Here's how the part is built. I have some questions about the finished solid (model axes, mm). Face numbers are marked on the shaded views. A direction names the side the tool comes from. Round coordinates to 2 decimals unless told otherwise and drop trailing zeros. Order: outer loops, then holes, each group sorted by start corner. A loop starts at its lowest first (then second) coordinate and runs counter-clockwise, first axis right, second up. Notation, with made-up numbers: (-16, -13) - (0, -13) arc R4 ccw to (0, -8) - close; hole circle Ø4 at (-7, -6.75). An arc over 180 degrees is marked (long way). One line per item, written item: value.
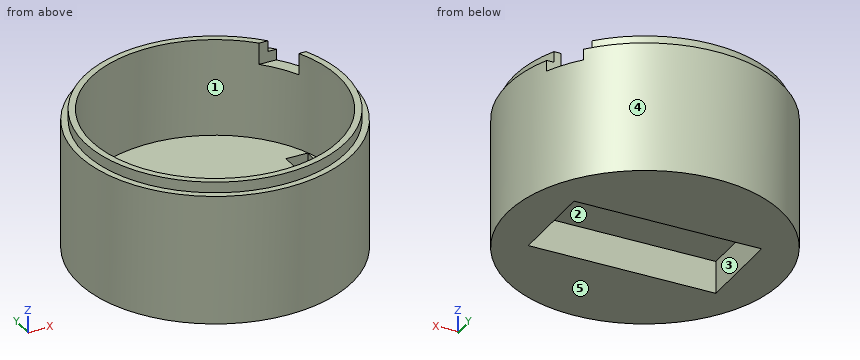
from build123d import *

# Parameters (mm, degrees)
F0_R      = 63
F0_R_2    = 60
F2_DEPTH  = 60
F1_R      = 60
F1_R_2    = 57
F3_DEPTH  = 65
F4_R      = 57
F5_DEPTH  = 60
F7_R      = 57
F8_DEPTH  = 40
F9_W      = 15
F9_H      = 10
F10_DEPTH = 279.5
F11_DEPTH = 71.5
F13_R     = 63
F14_DEPTH = 20
F15_W     = 86
F15_H     = 41
F16_DEPTH = 15
F17_W     = 27.3
F17_H     = 13
F18_DEPTH = 53
F20_DEPTH = 25


# Not quite as in the source:
# - a feature names something its author has since deleted; it is built from what else it names


with BuildPart() as f2:
    # F0 (on Top) → F2 (new body)
    with BuildSketch(Plane.XY):
        Circle(F0_R)
        Circle(F0_R_2, mode=Mode.SUBTRACT)
    extrude(amount=F2_DEPTH)

    # F1 (on Top) → F3 (join)
    with BuildSketch(Plane.XY):
        Circle(F1_R)
        Circle(F1_R_2, mode=Mode.SUBTRACT)
    extrude(amount=F3_DEPTH)

    # F4 (on Top) → F5 (join)
    with BuildSketch(Plane.XY):
        Circle(F4_R)
    extrude(amount=F5_DEPTH)

    # F7 (on offset) → F8 (cut)
    with BuildSketch(Plane.XY.offset(45)):
        Circle(F7_R)
    extrude(amount=-F8_DEPTH, mode=Mode.SUBTRACT)

    # F9 (on Right) → F10 (cut)
    with BuildSketch(Plane.YZ):
        with Locations((32.5, 60)):
            Rectangle(F9_W, F9_H)
    extrude(amount=F10_DEPTH, mode=Mode.SUBTRACT)

    # F1 (on Top) → F11 (cut)
    with BuildSketch(Plane.XY):
        Circle(F1_R_2)
    extrude(amount=F11_DEPTH, mode=Mode.SUBTRACT)

    # F13 (on Top) → F14 (join)
    with BuildSketch(Plane.XY):
        Circle(F13_R)
    extrude(amount=F14_DEPTH)

    # F15 (on Top) → F16 (cut)
    with BuildSketch(Plane.XY):
        Rectangle(F15_W, F15_H)
    extrude(amount=F16_DEPTH, mode=Mode.SUBTRACT)

    # F17 (on Right) → F18 (cut)
    with BuildSketch(Plane.YZ):
        with Locations((6.82, 8.5)):
            Rectangle(F17_W, F17_H)
    extrude(amount=F18_DEPTH, mode=Mode.SUBTRACT)

    # F19 (on offset) → F20 (cut)
    with BuildSketch(Plane.XY.offset(15)):
        Polygon((43, 20.47), (43, 0), (43, -6.83), (53, -6.83), (53, 20.47), align=None)
    extrude(amount=F20_DEPTH, mode=Mode.SUBTRACT)


solid = f2.part
Q1. If we section it at D-D, the plane z = 57: Please give me the cut outline in (x, y) (3 decimals), then the cut area to 3 significant figures.
Results list:
outline: (40.608, 40) - (48.672, 40) arc R63 ccw (long way) to (57.827, 25) - (51.225, 25) arc R57 cw (long way) to start
area: 2,150 mm²
Q2. We'd pull the mould along X, two halves only. Please class the marked faces 3, 4 and 5: released by +X, released by -X, zero draft, split by the parting line, or undercut.
Results list:
face 3: undercut
face 4: split by the parting line
face 5: zero draft
Q3. If we section it at C-C, the plane x = 0: Please give me the cut outline in (y, z).
Results list:
outline: (-63, 0) - (-20.5, 0) - (-20.5, 15) - (20.5, 15) - (20.5, 0) - (63, 0) - (63, 60) - (60, 60) - (60, 65) - (57, 65) - (57, 20) - (-57, 20) - (-57, 65) - (-60, 65) - (-60, 60) - (-63, 60) - close
Q4. If we section it at B-B, the plane y = 0: Please give me the cut outline in (x, z).
Results list:
outline: (-63, 0) - (-43, 0) - (-43, 15) - (43, 15) - (43, 20) - (-57, 20) - (-57, 65) - (-60, 65) - (-60, 60) - (-63, 60) - close; (43, 0) - (63, 0) - (63, 60) - (60, 60) - (60, 65) - (57, 65) - (57, 20) - (53, 20) - (53, 2) - (43, 2) - close
Q5. If I drill on line 1 along Y through (x, z) = (0, 41); line 2 along Z through (x, y) = (16.5, -41.5); line 3 along X through (y, z) = (-2, 56.5), over which ranges is the centre line in solid material (lowest first)?
Results list:
line 1: -63 to -57, 57 to 63
line 2: 0 to 20
line 3: -62.97 to -56.96, 56.96 to 62.97
Q6. Which directions (+Z, -Z, +X, -X, +Y, -Y) give clear straight access to the entire face, cutting with the end or side of a thin tool? Please do the marked faces 1 and 2.
Results list:
face 1: +Z
face 2: -Z
Q7. Will these pins go through, and if not, where does the flat tip stop? pin 1 (5 mm diameter, centred on x = 48.5, y = -19, fed in from +Z); pin 2 (12.5 mm diameter, centred on x = -18, y = -3, fed in from -Z); pin 3 (1 mm diameter, centred on x = 30.5, z = 23.5, fed in from -Y).
Results list:
pin 1: z = 20
pin 2: z = 15
pin 3: y = -55.4
